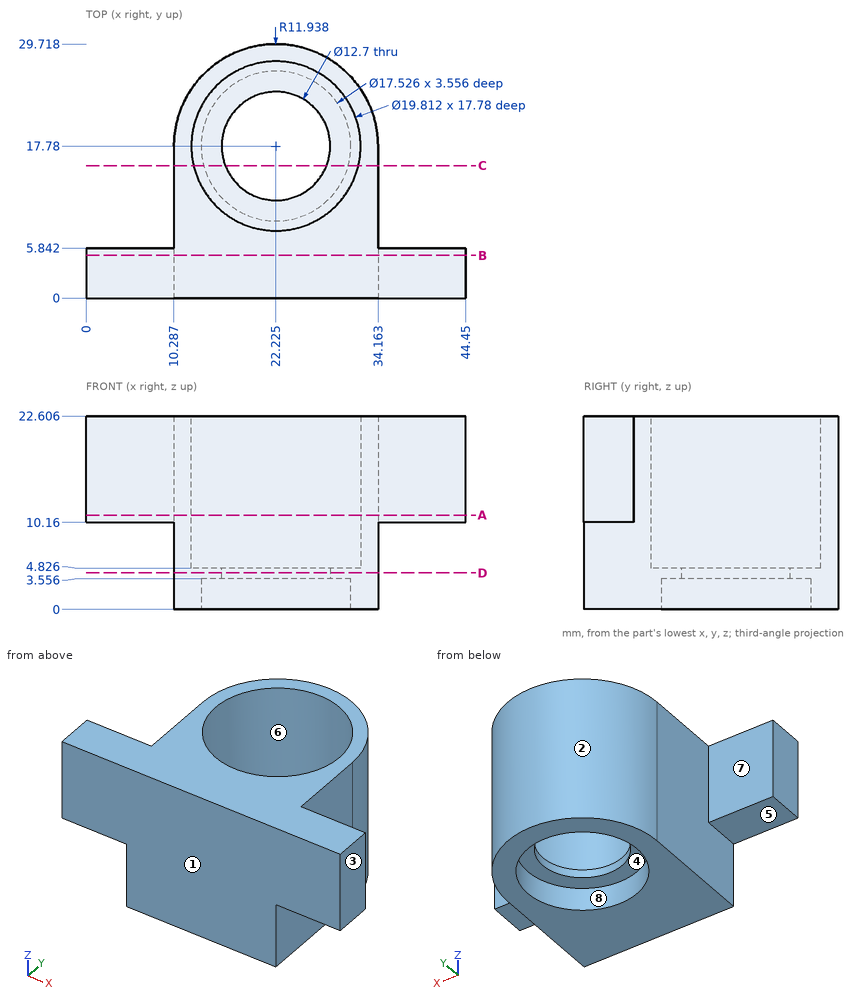
The figure shows three views and two pictorial views of one solid part (mm, origin at its lowest corner). Answer the questions. A direction names the side the tool comes from. Coordinates: 2 decimals unless noted, no trailing zeros. Order: outer loops, then holes, each group sorted by start corner. A loop starts at its lowest first (then second) coordinate and runs counter-clockwise, first axis right, second up.
Q1. A cutting plane is placed at A-A, the plane z = 11. Write down the section's boundary in (x, y) (3 decimals), and give its area (3 significant figures).
Q2. A cutting plane is placed at D-D, the plane z = 4.25. Write down the section's boundary in (x, y) (3 decimals), and give its area (3 significant figures).
Q3. A cutting plane is placed at B-B, the plane y = 5. Write down the section's boundary in (x, z), and give its area (3 significant figures).
Q4. For a pull along Y with two mould halves and no side action, classify the marked faces 1, 2, 3 and 4 as pulls with the +Y half, pulls with the -Y half, needs draft (parallel to the pull), parting line crosses it, or undercut.
Q5. A cutting plane is placed at C-C, the plane y = 15.5. Write down the section's boundary in (x, z), and give its area (3 significant figures).
Q6. Which of the six approach directions +Z, -Z, +X, -X, +Y, -Y give full straight-line access (tool end or side, diameter ignored) to the marked faces 5, 6, 7 and 8?
Q7. Given P1, Ø5, axis at y = 17, z = 8.5, coming from the +X side; P2, Ø2, axis at x = 27.5, y = 24.5, coming from the +Z side; P3, Ø11.5, axis at x = 5.5, z = 18.5, coming from the +Y side; P4, Ø12, axis at y = 3, z = 9.5, coming from the -X side, each flat-ended and moving along its own axis, determine where each tip first touches the part or whether it passes through.
Q8. Consider line 1 (X direction, y = 18.25, z = 5.5); line 2 (X direction, y = 9, z = 5); line 3 (Y direction, x = 19, z = 9.5). Determine where each line is inside the solid, lowest interval first.
Answers follow:
1. outline: (0, 0) - (44.45, 0) - (44.45, 5.842) - (34.163, 5.842) - (34.163, 17.78) arc R11.938 ccw to (10.287, 17.78) - (10.287, 5.842) - (0, 5.842) - close; hole circle Ø19.812 at (22.225, 17.78)
1. area: 460 mm2
2. outline: (10.287, 0) - (34.163, 0) - (34.163, 17.78) arc R11.938 ccw to (10.287, 17.78) - close; hole circle Ø12.7 at (22.225, 17.78)
2. area: 522 mm2
3. outline: (0, 10.16) - (10.29, 10.16) - (10.29, 0) - (34.16, 0) - (34.16, 10.16) - (44.45, 10.16) - (44.45, 22.61) - (0, 22.61) - close
3. area: 796 mm2
4. face 1: pulls with the -Y half
4. face 2: pulls with the +Y half
4. face 3: needs draft
4. face 4: undercut
5. outline: (10.29, 0) - (13.76, 0) - (13.76, 3.56) - (16.3, 3.56) - (16.3, 4.83) - (12.58, 4.83) - (12.58, 22.61) - (10.29, 22.61) - close; (28.15, 3.56) - (30.69, 3.56) - (30.69, 0) - (34.16, 0) - (34.16, 22.61) - (31.87, 22.61) - (31.87, 4.83) - (28.15, 4.83) - close
5. area: 122 mm2
6. face 5: -Z, -X, +Y, -Y
6. face 6: +Z
6. face 7: +Z, -Z, -X, +Y
6. face 8: -Z
7. P1: stops at x = 34.16
7. P2: stops at z = 4.83
7. P3: stops at y = 22.48
7. P4: stops at x = 0
8. line 1: x = 10.3 to 12.33, 32.12 to 34.15
8. line 2: x = 10.29 to 17.64, 26.81 to 34.16
8. line 3: y = 0 to 8.41, 27.15 to 29.27
